For this review, use the dimensioned drawing (mm, ordinates from the lowest corner) and the shaded views. Round coordinates to 2 decimals unless told otherwise and drop trailing zeros. Order: outer loops, then holes, each group sorted by start corner. A loop starts at its lowest first (then second) coordinate and runs counter-clockwise, first axis right, second up. Notation, with made-up numbers: M 81,5 L 109,5 A14 cw 109,15 Z; hole C -11.5,42 d8. An arc over 180 degrees is marked long. One line per item, written item: value. Start each with the question number.
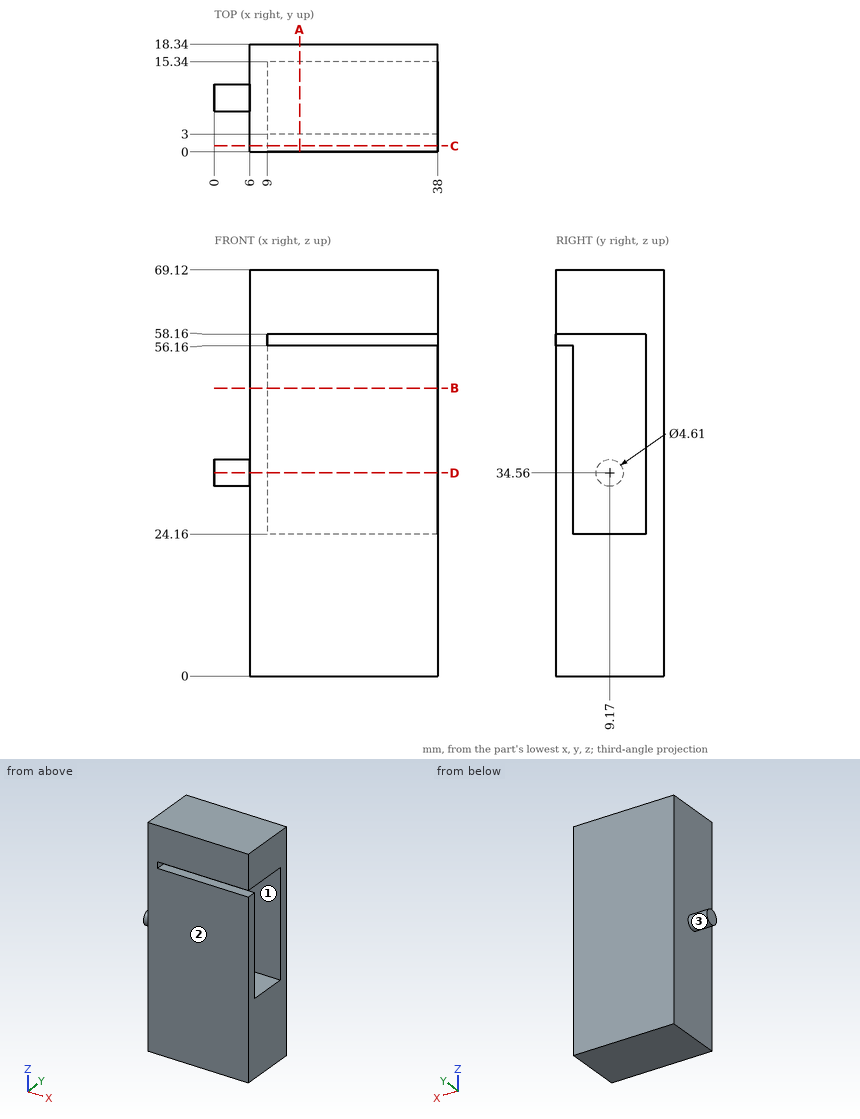
Item 1: The part is to be moulded in two halves that separate along Y. For the marked faces 1, 2 and 3, say which applies: pulls with the +Y half, pulls with the -Y half, needs draft (parallel to the pull), parting line crosses it, or undercut.
Item 2: Clearance check with flat-ended pins moving along their axes: P1, Ø4.5, axis at y = 6, z = 44.5, coming from the +X side; P2, Ø3, axis at y = 4, z = 49.5, coming from the -X side; P3, Ø4.5, axis at x = 19, y = 4.5, coming from the -Z side. State where each tip first meets the part, or that it passes through.
Item 3: Consider section D-D, the plane z = 34.56. Give the boundary of the cut face in (x, y) (3 decimals).
Item 4: Consider section C-C, the plane y = 1. Give the boundary of the cut face in (x, z).
Item 5: Consider section B-B, the plane z = 49. Give the boundary of the cut face in (x, y), then the cut area to 3 significant figures.
Item 6: Consider section A-A, the plane x = 14.5. Give the boundary of the cut face in (y, z).
Item 7: Wall thickness on L1, parallel to Z at x = 19, y = 7.75; L2, parallel to Y at x = 28.5, z = 37.5; L3, parallel to Z at x = 32.5, y = 1: over which ranges is each line inside the solid? List them lowest first.
Computed:
1. face 1: undercut
1. face 2: pulls with the -Y half
1. face 3: parting line crosses it
2. P1: stops at x = 9
2. P2: stops at x = 6
2. P3: stops at z = 0
3. outline: M 0,6.865 L 6,6.865 L 6,0 L 38,0 L 38,3 L 9,3 L 9,15.34 L 38,15.34 L 38,18.34 L 6,18.34 L 6,11.475 L 0,11.475 Z
4. outline: M 6,0 L 38,0 L 38,56.16 L 9,56.16 L 9,58.16 L 38,58.16 L 38,69.12 L 6,69.12 Z
5. outline: M 6,0 L 38,0 L 38,3 L 9,3 L 9,15.34 L 38,15.34 L 38,18.34 L 6,18.34 Z
5. area: 229 mm^2
6. outline: M 0,0 L 18.34,0 L 18.34,69.12 L 0,69.12 L 0,58.16 L 15.34,58.16 L 15.34,24.16 L 3,24.16 L 3,56.16 L 0,56.16 Z
7. L1: z = 0 to 24.16, 58.16 to 69.12
7. L2: y = 0 to 3, 15.34 to 18.34
7. L3: z = 0 to 56.16, 58.16 to 69.12
